Could you check a few things on this drawing? It's one solid part, dimensions in mm from its lowest x, y, z. Coordinates: 2 decimals unless noted, no trailing zeros. Order: outer loops, then holes, each group sorted by start corner. A loop starts at its lowest first (then second) coordinate and runs counter-clockwise, first axis right, second up.
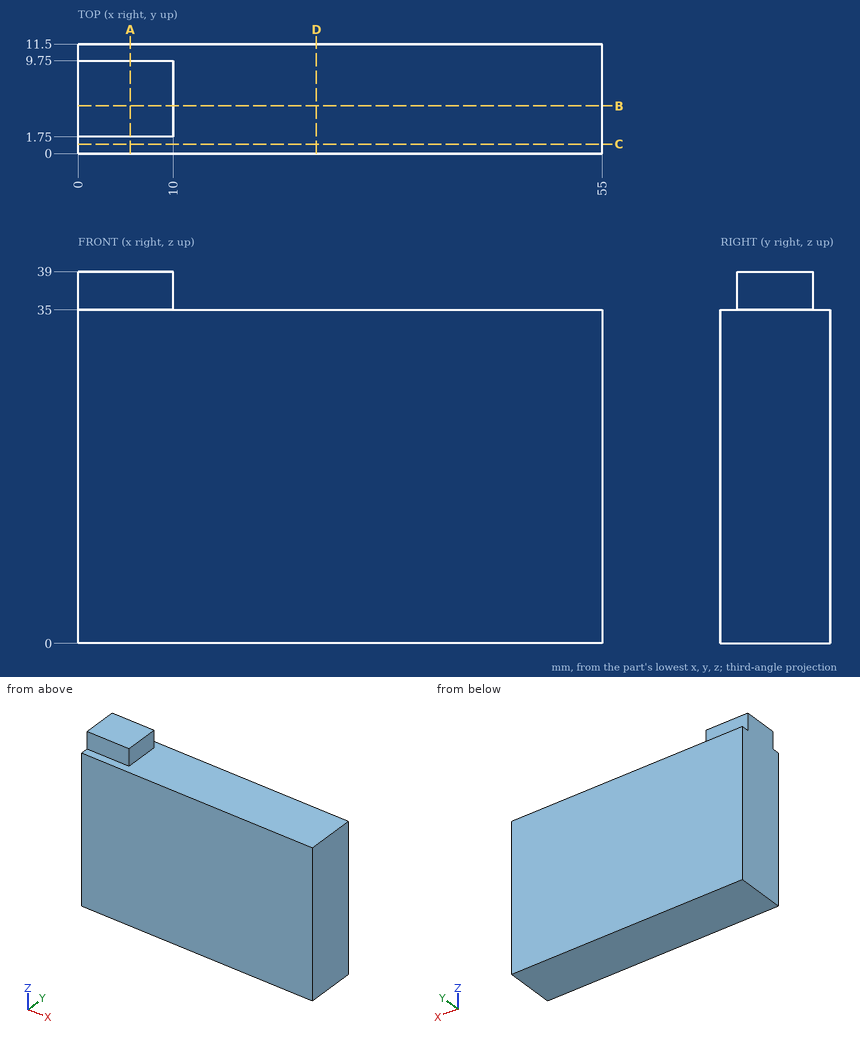
Item 1: Suppose I cut it at C-C (y = 1). List the corners of the cut face in (x, z) for me, and give its area (4 significant figures).
Item 2: Suppose I cut it at D-D (x = 25). List the corners of the cut face in (y, z) for me.
Item 3: I need wall thicknesses on line 1 (Z direction, x = 26.5, y = 3.25); line 2 (Y direction, x = 7.5, z = 37.5); line 3 (X direction, y = 3.5, z = 36.5). Which ranges of each line are inside material? Lowest first, please.
Item 4: Suppose I cut it at B-B (y = 5). List the corners of the cut face in (x, z) for me, and give its area (4 significant figures).
Item 5: Suppose I cut it at A-A (x = 5.5). List the corners of the cut face in (y, z) for me.
Item 6: For pin 1 Ø6 at (x, y) = (47, 2.5) entering from +Z; pin 2 Ø1.2 at (y, z) = (6, 37.5) entering from +X; pin 3 Ø1.2 at (x, z) = (7, 38) entering from -Y, each with a flat end and sliding along its axis, tell me the tip position at first contact or that it passes through.
Geometry results:
1. outline: (0, 0) - (55, 0) - (55, 35) - (0, 35) - close
1. area: 1,925 mm2
2. outline: (0, 0) - (11.5, 0) - (11.5, 35) - (0, 35) - close
3. line 1: z = 0 to 35
3. line 2: y = 1.75 to 9.75
3. line 3: x = 0 to 10
4. outline: (0, 0) - (55, 0) - (55, 35) - (10, 35) - (10, 39) - (0, 39) - close
4. area: 1,965 mm2
5. outline: (0, 0) - (11.5, 0) - (11.5, 35) - (9.75, 35) - (9.75, 39) - (1.75, 39) - (1.75, 35) - (0, 35) - close
6. pin 1: stops at z = 35
6. pin 2: stops at x = 10
6. pin 3: stops at y = 1.75
